The listing builds one solid part. Answer for the finished solid, in the listing's coordinates (mm). A direction names the side the tool comes from. Round coordinates to 2 decimals unless told otherwise and drop trailing zeros. Write each loop counter-clockwise with the first axis right and the second up, starting at its lowest first coordinate (ties: lowest second). Pieces come first, ordered by that corner, then holes. Notation, with made-up numbers: (-17.5, 12) - (14.5, 12) arc R22 cw to (14.5, 30) - close; hole circle Ø1 at (-38, -22.75). An arc over 180 degrees is marked (long way). Answer in a Markdown table with one row per item.
Autodesk Inventor part; units mm, degrees
ref_plane "YZ Plane" through (0, 0, 0) normal (1, 0, 0) x (0, 1, 0)
ref_plane "XZ Plane" through (0, 0, 0) normal (0, 1, 0) x (-1, 0, 0)
ref_plane "XY Plane" through (0, 0, 0) normal (0, 0, 1) x (1, 0, 0)
sketch "Sketch1" plane through (0, 0, 0) normal (0, 1, 0) x (-1, 0, 0)
  circle A0 centre (0, 38) radius 6.65
  circle A1 centre (0, -38) radius 6.65
  circle A2 centre (0, 38) radius 10
  circle A3 centre (0, -38) radius 10
  line L0 (6.65, 48) -> (12.65, 48)
  line L1 (12.65, 48) -> (12.65, -48)
  line L2 (12.65, -48) -> (6.65, -48)
  line L3 (6.65, -48) -> (6.65, 48)
  line L4 (12.65, 48) -> (0, 48)
  line L5 (12.65, -48) -> (0, -48)
  line L6 (0, 28) -> (6.65, 28)
  line L7 (0, -28) -> (6.65, -28)
  line L8 (0, 48) -> (0, -48)
  point P0 (0, 0)
  point P1 (0, 31.35)
  point P2 (0, -31.35)
  point P3 (0, -44.65)
  point P4 (6.65, -45.4684)
  point P5 (0, 44.65)
  dimension "d0" = 38
  dimension "d1" = 38
  dimension "d2" = 13.3
  dimension "d3" = 20
  dimension "d4" = 20
  dimension "d5" = 6
extrude "Extrusion1" add sketch "Sketch1" along normal blind 10 contours L3 A2 L8 A0 | L3 A2 | A0 L8 A2 L3 | L3 L6 A2 | A2 L3 L0 L1 L2 A3 | A2 L4 L3 | L7 L3 A3 | A3 L3 A1 L8 | L8 A1 L3 A3 | A3 L3 L5 | A3 L3
fillet "Fillet1" radius 5 4 edges at (-12.65, 5, 48) (-12.65, 5, -48) (-6.65, 5, -28) (-6.65, 5, 28)
sketch "Sketch2" plane through (0, 0, -44.65) normal (1, 0, 0) x (0, 0, -1)
  line L0 (0, 0) -> (3.35, 0)
  line L1 (3.35, 0) -> (3.35, 10)
  line L2 (0, 10) -> (3.35, 10)
  line L3 (0, 0) -> (0, 10)
  line L4 (-16.65, 0) -> (-13.3, 0)
  line L5 (-13.3, 0) -> (-13.3, 10)
  line L6 (-16.65, 10) -> (-13.3, 10)
  line L7 (-16.65, 0) -> (-16.65, 10)
  line L8 (-76, 0) -> (-72.65, 0)
  line L9 (-72.65, 0) -> (-72.65, 10)
  line L10 (-76, 10) -> (-72.65, 10)
  line L11 (-76, 0) -> (-76, 10)
  line L12 (-92.65, 0) -> (-89.3, 0)
  line L13 (-89.3, 0) -> (-89.3, 10)
  line L14 (-92.65, 10) -> (-89.3, 10)
  line L15 (-92.65, 0) -> (-92.65, 10)
  point P0 (-44.65, 0)
extrude "Extrusion2" add sketch "Sketch2" along normal blind 6
properties part number "Base"
(1) Section D-D (z = 38) is taken. Give the vertices of the cut face in (x, y).
Checked values:
| item | result |
|---|---|
| outline | (-12.65, 0) - (-6.65, 0) - (-6.65, 10) - (-12.65, 10) - close |
(2) For a pull along Z with two mould halves and no side action, classify faces 3 (the flat face through (-7, 10, 1)), 4 (the cylindrical face through (-11.22, 5.07, 46.5)), 5 (the cylindrical face through (-5.22, 5.07, 26.5)) as pulls with the +Z half, pulls with the -Z half, needs draft (parallel to the pull), parting line crosses it, or undercut.
Checked values:
| item | result |
|---|---|
| face 3 | needs draft |
| face 4 | pulls with the +Z half |
| face 5 | undercut |
(3) Section B-B (y = 4.75) is taken. Give the vertices of the cut face in (x, z).
Checked values:
| item | result |
|---|---|
| outline | (-12.65, -43) arc R5 ccw to (-7.65, -48) - (6, -48) - (6, -44.65) - (0, -44.65) arc R6.65 cw to (0, -31.35) - (6, -31.35) - (6, -28) - (-1.65, -28) arc R5 cw to (-6.65, -23) - (-6.65, 23) arc R5 cw to (-1.65, 28) - (6, 28) - (6, 31.35) - (0, 31.35) arc R6.65 cw to (0, 44.65) - (6, 44.65) - (6, 48) - (-7.65, 48) arc R5 ccw to (-12.65, 43) - close |
(4) Flat-ended cylindrical pins translate along their axes: pin 1 (3 mm diameter, centred on y = 3, z = 5.5, fed in from +X); pin 2 (6 mm diameter, centred on y = 1.5, z = -35, fed in from +X). Find the tip coordinate at first contact, or state that the pin passes through.
Checked values:
| item | result |
|---|---|
| pin 1 | stops at x = -6.65 |
| pin 2 | stops at x = -2.87 |
(5) Find the intervals of material crossed by line 1 (Z direction, x = 4, y = 6.5); line 2 (Z direction, x = -3.5, y = 2.75); line 3 (X direction, y = 4.25, z = 4), in increasing order.
Checked values:
| item | result |
|---|---|
| line 1 | z = -48 to -44.65, -31.35 to -28, 28 to 31.35, 44.65 to 48 |
| line 2 | z = -48 to -43.65, -32.35 to -27.65, 27.65 to 32.35, 43.65 to 48 |
| line 3 | x = -12.65 to -6.65 |
(6) For faces 1 (the flat face through (-6.65, 5, 0)), 2 (the flat face through (6, 5, 46)), determine the directions among +Z, -Z, +X, -X, +Y, -Y from which every point of the face is accessible in a straight line to the end or side of a thin tool.
Checked values:
| item | result |
|---|---|
| face 1 | +X, +Y, -Y |
| face 2 | +Z, -Z, +X, +Y, -Y |
(7) Section A-A (x = 1.25) is taken. Give the vertices of the cut face in (y, z).
Checked values:
| item | result |
|---|---|
| outline | (0, -48) - (10, -48) - (10, -44.65) - (0, -44.65) - close; (0, -31.35) - (10, -31.35) - (10, -28) - (0, -28) - close; (0, 28) - (10, 28) - (10, 31.35) - (0, 31.35) - close; (0, 44.65) - (10, 44.65) - (10, 48) - (0, 48) - close |
(8) Section C-C (x = -3) is taken. Give the vertices of the cut face in (y, z).
Checked values:
| item | result |
|---|---|
| outline | (0, -48) - (10, -48) - (10, -43.93) - (0, -43.93) - close; (0, -32.07) - (10, -32.07) - (10, -27.81) - (0, -27.81) - close; (0, 27.81) - (10, 27.81) - (10, 32.07) - (0, 32.07) - close; (0, 43.93) - (10, 43.93) - (10, 48) - (0, 48) - close |
